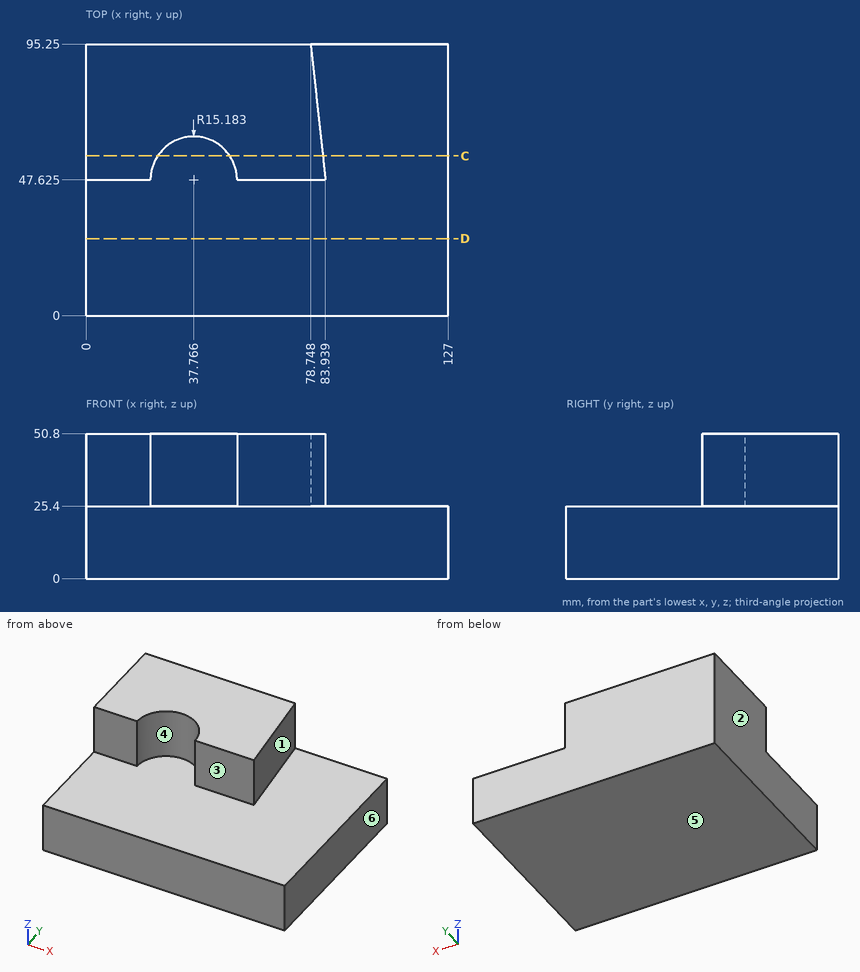
Study the drawing (mm; zero at the part's minimum x, y, z) and answer. A direction names the side the tool comes from. Coordinates: 2 decimals unless noted, no trailing zeros. Write each loop counter-clockwise with the first axis right and the second up, starting at its lowest first coordinate (ties: lowest second). Pieces come first, ordered by that corner, then holes. Notation, with made-up numbers: (27.25, 55.25) - (41.25, 55.25) arc R23 ccw to (41.25, 79.25) - close; hole circle Ø2 at (-11.75, -34.75). An arc over 180 degrees is marked (long way). One line per question, with ' | ' between items.
1) For the marked faces 1, 2 and 3, determine the directions among +Z, -Z, +X, -X, +Y, -Y from which every point of the face is accessible in a straight line to the end or side of a thin tool.
Checks:
face 1: +Z, +X, +Y | face 2: +Z, -Z, -X, +Y, -Y | face 3: +Z, +X, -X, -Y
2) Consider probe 1 along Z at (x, y) = (73, 13); probe 2 along X at (y, z) = (56.5, 44) (1 decimal); probe 3 along X at (y, z) = (58.5, 32) (1 decimal). Determine where each line is inside the solid, lowest interval first. Write a range as [from, to].
Checks:
probe 1: [0, 25.4] | probe 2: [0, 25.4], [50.1, 83] | probe 3: [0, 27.2], [48.4, 82.8]
3) Flat-ended cylindrical pins translate along their axes: P1, Ø1, axis at x = 108, y = 26.5, coming from the +Z side; P2, Ø12.5, axis at x = 65.5, z = 38, coming from the -Y side (1 decimal); P3, Ø2, axis at x = 49.5, z = 40.5, coming from the -Y side (1 decimal). Find the tip coordinate at first contact, or state that the pin passes through.
Checks:
P1: z = 25.4 | P2: y = 47.6 | P3: y = 55.9
4) Find section D-D, the plane y = 27. Determine the outline of the cut face in (x, z), and give its area (3 significant figures).
Checks:
outline: (0, 0) - (127, 0) - (127, 25.4) - (0, 25.4) - close | area: 3,230 mm2
5) The mould has two halves that part along X. Classify the marked faces 4, 5 and 6: +X half, -X half, draft (parallel to the pull), parting line (faces both ways), or undercut.
Checks:
face 4: undercut | face 5: draft | face 6: +X half
6) Find section C-C, the plane y = 56. Determine the outline of the cut face in (x, z) (1 decimal), and give its area (3 significant figures).
Checks:
outline: (0, 0) - (127, 0) - (127, 25.4) - (83, 25.4) - (83, 50.8) - (50.4, 50.8) - (50.4, 25.4) - (25.1, 25.4) - (25.1, 50.8) - (0, 50.8) - close | area: 4,690 mm2
